from build123d import *

# Parameters (mm, degrees)
SKETCH_1_W               = 20
SKETCH_1_H               = 20
EXTRUDE_1_DEPTH          = 595.07
CUT_EXTRUDE_1_DEPTH      = 595.07
CUT_EXTRUDE_2_DEPTH      = 596.741810603
CUT_EXTRUDE_2_DEPTH_BACK = 596.741810603
SKETCH_3_R               = 2
SKETCH_4_R               = 2.15
CUT_EXTRUDE_3_DEPTH      = 20
SKETCH_5_R               = 2.15
SKETCH_5_R_2             = 2.1
CUT_EXTRUDE_4_DEPTH      = 137
SKETCH_9_R               = 2.1
CUT_EXTRUDE_5_DEPTH      = 32


with BuildPart() as part:
    # 草图1 → 凸台-拉伸1 (new body)
    with BuildSketch(Plane.XY):
        with Locations((10, 10)):
            Rectangle(SKETCH_1_W, SKETCH_1_H)
    extrude(amount=EXTRUDE_1_DEPTH)

    # 草图2 → 切除-拉伸1 (cut)
    with BuildSketch(Plane(origin=(0, 20, 0), x_dir=(1, 0, 0), z_dir=(0, 1, 0))):
        Polygon((0, -595.07), (20, -560.428983849), (20, -595.07), align=None)
    extrude(amount=-CUT_EXTRUDE_1_DEPTH, mode=Mode.SUBTRACT)

    # 草图3 → 切除-拉伸2 (cut, two sides: drawn at the far end of the back side and taken through both)
    with BuildSketch(Plane(origin=(0, 20, 0), x_dir=(1, 0, 0), z_dir=(0, 1, 0)).offset(-CUT_EXTRUDE_2_DEPTH_BACK)):
        with Locations(Location((10, -10, 0), (0, 0, 270))):
            Circle(SKETCH_3_R)
        with Locations(Location((10, -30, 0), (0, 0, 270))):
            Circle(SKETCH_3_R)
        with Locations(Location((10, -66.35, 0), (0, 0, 270))):
            Circle(SKETCH_3_R)
        with Locations(Location((10, -86.35, 0), (0, 0, 270))):
            Circle(SKETCH_3_R)
        with Locations(Location((10, -106.35, 0), (0, 0, 270))):
            Circle(SKETCH_3_R)
    extrude(amount=CUT_EXTRUDE_2_DEPTH + CUT_EXTRUDE_2_DEPTH_BACK, mode=Mode.SUBTRACT)

    # 草图4 → 切除-拉伸3 (cut)
    with BuildSketch(Plane(origin=(0, 20, 0), x_dir=(1, 0, 0), z_dir=(0, 1, 0))):
        with Locations(Location((10, -544.338983849, 0), (0, 0, 270))):
            Circle(SKETCH_4_R)
        with Locations(Location((10, -559.338983849, 0), (0, 0, 270))):
            Circle(SKETCH_4_R)
        with Locations(Location((10, -514.338983849, 0), (0, 0, 270))):
            Circle(SKETCH_4_R)
        with Locations(Location((10, -494.338983849, 0), (0, 0, 270))):
            Circle(SKETCH_4_R)
    extrude(amount=-CUT_EXTRUDE_3_DEPTH, mode=Mode.SUBTRACT)

    # 草图5 → 切除-拉伸4 (cut)
    with BuildSketch(Plane(origin=(0, 20, 0), x_dir=(1, 0, 0), z_dir=(0, 1, 0))):
        with Locations(Location((10, -205, 0), (0, 0, 270))):
            Circle(SKETCH_5_R)
        with Locations(Location((10, -221, 0), (0, 0, 270))):
            Circle(SKETCH_5_R_2)
        with Locations(Location((10, -310, 0), (0, 0, 270))):
            Circle(SKETCH_5_R_2)
        with Locations(Location((10, -290, 0), (0, 0, 270))):
            Circle(SKETCH_5_R_2)
        with Locations(Location((10, -330, 0), (0, 0, 270))):
            Circle(SKETCH_5_R_2)
    extrude(amount=-CUT_EXTRUDE_4_DEPTH, mode=Mode.SUBTRACT)

    # 草图9 → 切除-拉伸5 (cut)
    with BuildSketch(Plane(origin=(20, 0, 0), x_dir=(0, 0, -1), z_dir=(1, 0, 0))):
        with Locations((-467.690453805, 10)):
            Circle(SKETCH_9_R)
        with Locations((-487.690453805, 10)):
            Circle(SKETCH_9_R)
        with Locations((-447.690453805, 10)):
            Circle(SKETCH_9_R)
        with Locations((-357.460423925, 10)):
            Circle(SKETCH_9_R)
        with Locations((-377.460423925, 10)):
            Circle(SKETCH_9_R)
        with Locations((-337.460423925, 10)):
            Circle(SKETCH_9_R)
    extrude(amount=-CUT_EXTRUDE_5_DEPTH, mode=Mode.SUBTRACT)


solid = part.part
The model under review builds one solid part; all positions refer to its coordinate system, in mm. Give positions to 0.01 mm unless a question says otherwise; leave off trailing zeros. Write each loop counter-clockwise with the first axis right and the second up, starting at its lowest first coordinate (ties: lowest second). Pieces come first, ordered by that corner, then holes. Notation, with made-up numbers: M -16.5,-28 L 19.5,-28 A21 ccw 19.5,-10 Z; hole C 38,55 d2. An arc over 180 degrees is marked long. One line per question, with ' | ' between items. Start each with the question number.
Item 1: For pin 1 (2 mm diameter, centred on x = 15, y = 15.5, fed in from +Z); pin 2 (12 mm diameter, centred on x = 14.5, y = 18, fed in from +Z); pin 3 (5 mm diameter, centred on x = 3, y = 17.5, fed in from +Z), all flat-tipped, find the tip position at first contact; note any pin that passes through.
Item 2: We need section B-B on x = 3.5. Write out the cut boundary in (y, z), plus the area to 3 significant figures.
Item 3: Wall thickness on line 1 (X direction, y = 10.5, z = 10); line 2 (X direction, y = 11.5, z = 310); line 3 (Z direction, x = 1.75, y = 17): over which ranges is each line inside the solid? List them lowest first. Write a range as from..to.
Item 4: We need section A-A on y = 16.75. Give the number of separate pieces and of enclosed holes in the cut face, plus the area to 3 significant figures.
Results found:
1) pin 1: stops at z = 570.82 | pin 2: stops at z = 580.35 | pin 3: stops at z = 594.2
2) outline: M 0,0 L 20,0 L 20,589.01 L 0,589.01 Z; hole C 10,337.46 d4.2; hole C 10,357.46 d4.2; hole C 10,377.46 d4.2; hole C 10,447.69 d4.2; hole C 10,467.69 d4.2; hole C 10,487.69 d4.2 | area: 11,700 mm2
3) line 1: x = 0..8, 12..20 | line 2: x = 0..7.9, 12.1..20 | line 3: z = 0..592.04
4) separate pieces: 1 | enclosed holes: 14 | area: 11,400 mm2
